from build123d import *


with BuildPart() as part:
    # 草图1 → 旋转1 (revolve)
    with BuildSketch(Plane.XY, mode=Mode.PRIVATE) as revolve_1_sk:
        Polygon((0, 30), (1, 30), (1, 17), (1, 0), (10.2, 0), (10.2, 17), (10.2, 24.78), (33.6, 28.8226), (33.6, 30), (15.2, 30), (15.2, 31), (9.2, 31), (9.2, 30), (7.2, 30), (7.2, 46), (0, 46), align=None)
    revolve(revolve_1_sk.sketch.rotate(Axis((0, 0, 0), (1, 0, 0)), 90), axis=Axis((0, 0, 0), (1, 0, 0)))


solid = part.part
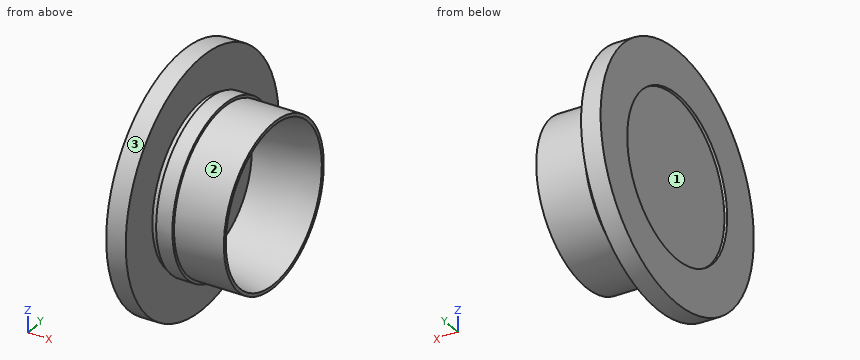
For this review, take the finished solid that the model builds, in its own axes (mm). Face numbers are marked on the shaded views. A direction names the side the tool comes from. Coordinates: 2 decimals unless noted, no trailing zeros. Order: outer loops, then holes, each group sorted by start corner. A loop starts at its lowest first (then second) coordinate and runs counter-clockwise, first axis right, second up. Notation, with made-up numbers: (22.25, 53) -> (40.25, 53) arc R15 cw to (40.25, 69) -> close; hole circle Ø10 at (63.5, 20). An arc over 180 degrees is marked (long way). Return JSON: item names as keys, results as strings.
1. We need section C-C on x = 5. Write out the cut boundary in (y, z).
Answer block:
{"outline": "circle Ø92 at (0, 0)"}
2. We need section D-D on x = 31. Write out the cut boundary in (y, z), and give its area (3 significant figures).
Answer block:
{"outline": "circle Ø60 at (0, 0); hole circle Ø56.75 at (0, 0)", "area": "298 mm²"}
3. We need section A-A on z = 0. Write out the cut boundary in (x, y).
Answer block:
{"outline": "(0, -46) -> (7.2, -46) -> (7.2, -30) -> (9.2, -30) -> (9.2, -31) -> (15.2, -31) -> (15.2, -30) -> (33.6, -30) -> (33.6, -28.82) -> (10.2, -24.78) -> (10.2, 24.78) -> (33.6, 28.82) -> (33.6, 30) -> (15.2, 30) -> (15.2, 31) -> (9.2, 31) -> (9.2, 30) -> (7.2, 30) -> (7.2, 46) -> (0, 46) -> (0, 30) -> (1, 30) -> (1, -30) -> (0, -30) -> close"}
4. Machinability: for the marked faces 1, 2 and 3, which of the approach directions +Z, -Z, +X, -X, +Y, -Y give a long, thin tool a straight path to every point of the face, cutting with its end or side? Answer none if there is none.
Answer block:
{"face 1": "-X", "face 2": "+X", "face 3": "+X, -X"}
5. For line 1 (Y direction, x = 0.4, z = 0); line 2 (X direction, y = -17.5, z = 9); line 3 (X direction, y = -14.5, z = 30.5), list the stretches that pass through material, from the lowest coordinate up. Write a range as from..to.
Answer block:
{"line 1": "-46..-30, 30..46", "line 2": "1..10.2", "line 3": "0..7.2"}
6. For pin 1 Ø3 at (x, z) = (4.5, 33) entering from +Y; pin 2 Ø8 at (x, z) = (6, -35) entering from -Y; pin 3 Ø2 at (x, y) = (4, -24) entering from +Z, all flat-tipped, find the tip position at first contact; note any pin that passes through.
Answer block:
{"pin 1": "y = 33.52", "pin 2": "y = -33.99", "pin 3": "z = 39.84"}
